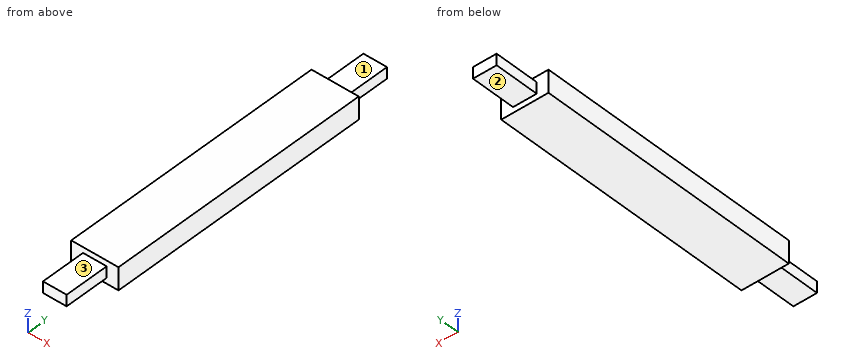
from build123d import *

# Parameters (mm, degrees)
SKETCH004_W     = 95
SKETCH004_H     = 720
PAD002_DEPTH    = 45
SKETCH014_W     = 95
SKETCH014_H     = 90
POCKET008_DEPTH = 11.25
SKETCH015_W     = 95
SKETCH015_H     = 90
POCKET009_DEPTH = 11.25
SKETCH016_W     = 23.75
SKETCH016_H     = 90
POCKET010_DEPTH = 11.25
SKETCH017_W     = 23.75
SKETCH017_H     = 90
POCKET011_DEPTH = 11.25
SKETCH018_W     = 23.75
SKETCH018_H     = 90
POCKET012_DEPTH = 11.25
SKETCH019_W     = 23.75
SKETCH019_H     = 90
POCKET013_DEPTH = 11.25


with BuildPart() as part:
    # Sketch004 → Pad002 (new body)
    with BuildSketch(Plane.XY):
        with Locations((47.5, 360)):
            Rectangle(SKETCH004_W, SKETCH004_H)
    extrude(amount=-PAD002_DEPTH)

    # Sketch014 (on Face5 of Pad002) → Pocket008 (cut)
    with BuildSketch(Plane.XY):
        with Locations((47.5, 45)):
            Rectangle(SKETCH014_W, SKETCH014_H)
        with Locations((47.5, 675)):
            Rectangle(SKETCH014_W, SKETCH014_H)
    extrude(amount=-POCKET008_DEPTH, mode=Mode.SUBTRACT)

    # Sketch015 (on Face4 of Pocket008) → Pocket009 (cut)
    with BuildSketch(Plane(origin=(0, 0, -45), x_dir=(1, 0, 0), z_dir=(0, 0, -1))):
        with Locations((47.5, -45)):
            Rectangle(SKETCH015_W, SKETCH015_H)
        with Locations((47.5, -675)):
            Rectangle(SKETCH015_W, SKETCH015_H)
    extrude(amount=-POCKET009_DEPTH, mode=Mode.SUBTRACT)

    # Sketch016 (on Face9 of Pocket009) → Pocket010 (cut)
    with BuildSketch(Plane.XY.offset(-11.25)):
        with Locations((11.875, 45)):
            Rectangle(SKETCH016_W, SKETCH016_H)
        with Locations((83.125, 45)):
            Rectangle(SKETCH016_W, SKETCH016_H)
    extrude(amount=-POCKET010_DEPTH, mode=Mode.SUBTRACT)

    # Sketch017 (on Face11 of Pocket010) → Pocket011 (cut)
    with BuildSketch(Plane(origin=(0, 0, -33.75), x_dir=(1, 0, 0), z_dir=(0, 0, -1))):
        with Locations((83.125, -45)):
            Rectangle(SKETCH017_W, SKETCH017_H)
        with Locations((11.875, -45)):
            Rectangle(SKETCH017_W, SKETCH017_H)
    extrude(amount=-POCKET011_DEPTH, mode=Mode.SUBTRACT)

    # Sketch018 (on Face5 of Pocket011) → Pocket012 (cut)
    with BuildSketch(Plane.XY.offset(-11.25)):
        with Locations((83.125, 675)):
            Rectangle(SKETCH018_W, SKETCH018_H)
        with Locations((11.875, 675)):
            Rectangle(SKETCH018_W, SKETCH018_H)
    extrude(amount=-POCKET012_DEPTH, mode=Mode.SUBTRACT)

    # Sketch019 (on Face3 of Pocket012) → Pocket013 (cut)
    with BuildSketch(Plane(origin=(0, 0, -33.75), x_dir=(1, 0, 0), z_dir=(0, 0, -1))):
        with Locations((11.875, -675)):
            Rectangle(SKETCH019_W, SKETCH019_H)
        with Locations((83.125, -675)):
            Rectangle(SKETCH019_W, SKETCH019_H)
    extrude(amount=-POCKET013_DEPTH, mode=Mode.SUBTRACT)


solid = part.part
Here's how the part is built. I have some questions about the finished solid (model axes, mm). Face numbers are marked on the shaded views. A direction names the side the tool comes from. Coordinates: 2 decimals unless noted, no trailing zeros. Order: outer loops, then holes, each group sorted by start corner. A loop starts at its lowest first (then second) coordinate and runs counter-clockwise, first axis right, second up.
Item 1: If we section it at C-C on x = 15.5: List the corners of the cut face in (y, z) for me.
Result sheet:
outline: (90, -45) - (630, -45) - (630, 0) - (90, 0) - close
Item 2: For the marked faces 1, 2 and 3, which set-ups out of +Z, -Z, +X, -X, +Y, -Y let a thin tool reach every point of the face, with its end or its side?
Result sheet:
face 1: +Z, +X, -X, +Y
face 2: -Z, +X, -X, +Y
face 3: +Z, +X, -X, -Y
Item 3: I need wall thicknesses on line 1 (Z direction, x = 38, y = 66.5); line 2 (Y direction, x = 7.5, z = -23.5); line 3 (X direction, y = 45.5, z = -12). Which ranges of each line are inside material? Lowest first, please.
Result sheet:
line 1: z = -33.75 to -11.25
line 2: y = 90 to 630
line 3: x = 23.75 to 71.25
Item 4: If we section it at B-B on y = 67: List the corners of the cut face in (x, z) for me, plus the area to 3 significant figures.
Result sheet:
outline: (23.75, -33.75) - (71.25, -33.75) - (71.25, -11.25) - (23.75, -11.25) - close
area: 1,070 mm2
Item 5: If we section it at A-A on z = -23.5: List the corners of the cut face in (x, y) for me.
Result sheet:
outline: (0, 90) - (23.75, 90) - (23.75, 0) - (71.25, 0) - (71.25, 90) - (95, 90) - (95, 630) - (71.25, 630) - (71.25, 720) - (23.75, 720) - (23.75, 630) - (0, 630) - close
Item 6: For P1, Ø7, axis at y = 696.5, z = -20.5, coming from the -X side; P2, Ø24, axis at x = 56.5, y = 54, coming from the +Z side; P3, Ø24, axis at x = 39.5, y = 667.5, coming from the -Z side, each with a flat end and sliding along its axis, tell me the tip position at first contact or that it passes through.
Result sheet:
P1: stops at x = 23.75
P2: stops at z = -11.25
P3: stops at z = -33.75
